Check sheet for the drawn part. Datum: minimum x, y, z corner. Units: mm. Coordinates: 2 decimals unless noted, no trailing zeros. Order: outer loops, then holes, each group sorted by start corner. A loop starts at its lowest first (then second) coordinate and runs counter-clockwise, first axis right, second up. Notation, with made-up numbers: M 68.25,64.25 L 109.25,64.25 A12 ccw 109.25,71.25 Z; hole C -8,-37 d5. An arc over 180 degrees is marked long. Use one line per item in the form item = value. Start each with the question number.
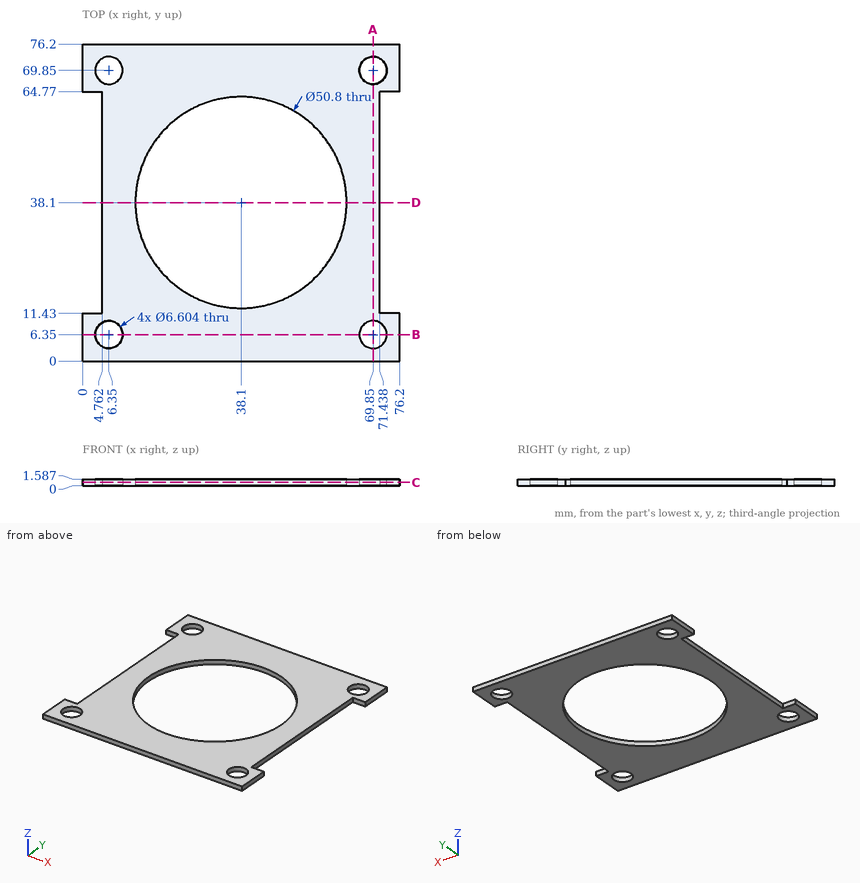
1. Cross-section at C-C on z = 0.8. Give the number of separate pieces and of enclosed holes in the cut face.
2. Material ranges on line 1 along X through (y, z) = (38, 1); line 2 along Y through (x, z) = (38.1, 1); line 3 along X through (y, z) = (69, 1.55), recorded low to high.
3. Cross-section at D-D on y = 38.1. Enter the section's corners in (x, z), and give its area (3 significant figures).
4. Cross-section at A-A on x = 69.85. Enter the section's corners in (y, z).
5. Depth check by flat-ended pin: P1, Ø0.8, axis at y = 46, z = 1, coming from the -X side; P2, Ø6, axis at x = 69.85, y = 69.85, coming from the -Z side. Enter the tip coordinate at first touch or a pass-through.
Final values:
q1.separate_pieces = 1
q1.enclosed_holes = 5
q2.line_1 = 4.76 to 12.7, 63.5 to 71.44
q2.line_2 = 0 to 12.7, 63.5 to 76.2
q2.line_3 = 0 to 3.16, 9.54 to 66.66, 73.04 to 76.2
q3.outline = M 4.76,0 L 12.7,0 L 12.7,1.59 L 4.76,1.59 Z; M 63.5,0 L 71.44,0 L 71.44,1.59 L 63.5,1.59 Z
q3.area = 25.2 mm2
q4.outline = M 0,0 L 3.05,0 L 3.05,1.59 L 0,1.59 Z; M 9.65,0 L 66.55,0 L 66.55,1.59 L 9.65,1.59 Z; M 73.15,0 L 76.2,0 L 76.2,1.59 L 73.15,1.59 Z
q5.P1 = 4.76
q5.P2 = through
